The drawing under review shows one solid part. Ordinate dimensions are in mm from its lowest x, y, z. Coordinates: 2 decimals unless noted, no trailing zeros. Write each loop counter-clockwise with the first axis right and the second up, starting at its lowest first coordinate (ties: lowest second). Pieces come first, ordered by that corner, then holes. Notation, with made-up numbers: (-3.75, 42.5) -> (10.25, 42.5) arc R14 cw to (10.25, 56.5) -> close; hole circle Ø2 at (43.25, 77). An arc over 180 degrees is marked (long way). One line per question, with ' | ' between items. Start each with the question number.
Q1. For P1, Ø3, axis at x = 152.654, z = 114.3, coming from the +Y side; P2, Ø6, axis at x = 355.6, z = 75.946, coming from the +Y side, all flat-tipped, find the tip position at first contact; note any pin that passes through.
Q2. Add section A-A on z = 68. State the section outline as (x, y) points, and give its area (3 significant figures).
Q3. Wall thickness on probe 1 along X at (y, z) = (3, 114.3); probe 2 along X at (y, z) = (0.5, 62); probe 3 along Z at (x, y) = (97, 4.5) (1 decimal): over which ranges is each line inside the solid? List them lowest first.
Q4. Draft analysis for pull direction Y (two halves, no side actions). For the marked faces 1 and 2, state which applies: pulls with the +Y half, pulls with the -Y half, needs draft (parallel to the pull), parting line crosses it, or undercut.
Q5. Add section C-C on y = 1.5. Give the number of separate pieces and of enclosed holes in the cut face, and give its area (3 significant figures).
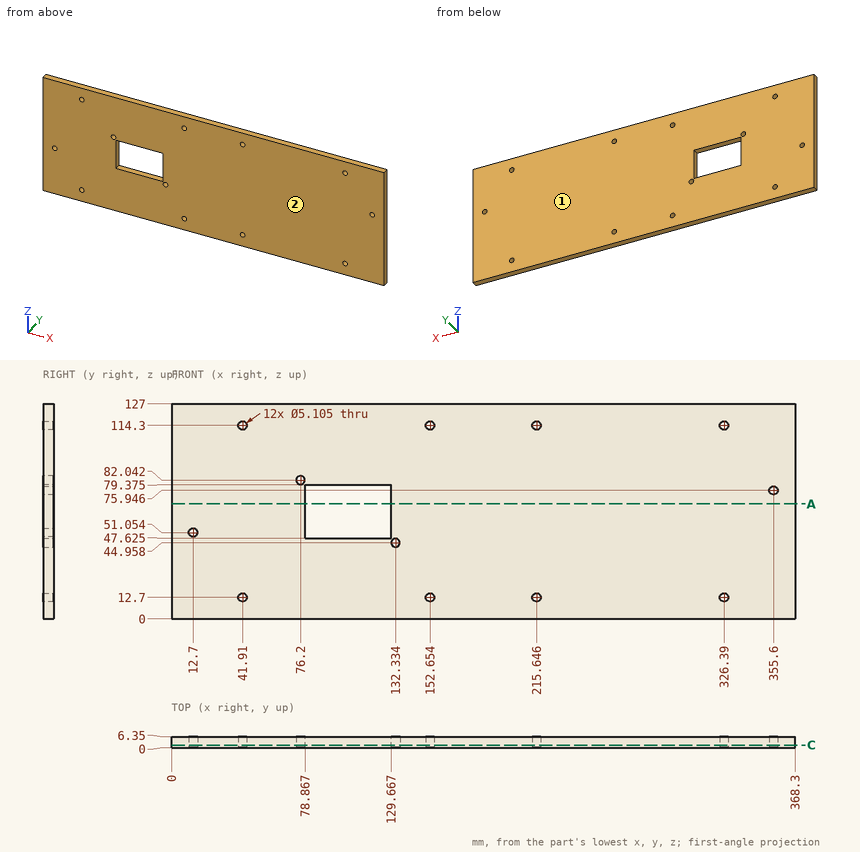
Output values:
1) P1: passes through | P2: stops at y = 6.35
2) outline: (0, 0) -> (78.87, 0) -> (78.87, 6.35) -> (0, 6.35) -> close; (129.67, 0) -> (368.3, 0) -> (368.3, 6.35) -> (129.67, 6.35) -> close | area: 2,020 mm2
3) probe 1: x = 0 to 39.36, 44.46 to 150.1, 155.21 to 213.09, 218.2 to 323.84, 328.94 to 368.3 | probe 2: x = 0 to 78.87, 129.67 to 368.3 | probe 3: z = 0 to 47.6, 79.4 to 127
4) face 1: pulls with the +Y half | face 2: pulls with the -Y half
5) separate pieces: 1 | enclosed holes: 13 | area: 44,900 mm2
